```python
from build123d import *

# Parameters (mm, degrees)
BOSS_EXTRUDE1_DEPTH = 22.5
SKETCH2_W           = 5
SKETCH2_H           = 5
CUT_EXTRUDE1_DEPTH  = 10


with BuildPart() as part:
    # Sketch1 → Boss-Extrude1 (new, symmetric)
    with BuildSketch(Plane.XY):
        with BuildLine():
            Line((1.939814393, 10.4209942), (1.904028006, 10.276656915))
            ThreePointArc((1.904028006, 10.276656915), (1.428480454, 9.568373768), (0.609305018, 9.330125797))
            ThreePointArc((0.609305018, 9.330125797), (-0.439609364, 9.339659716), (-1.482990759, 9.231643321))
            ThreePointArc((-1.482990759, 9.231643321), (-2.320923107, 9.391892722), (-2.860897269, 10.052376178))
            Line((-2.860897269, 10.052376178), (-2.910083052, 10.192713899))
            ThreePointArc((-2.910083052, 10.192713899), (-4.572008101, 10.932485624), (-5.212501917, 9.229833356))
            Line((-5.212501917, 9.229833356), (-5.14713766, 9.096261535))
            ThreePointArc((-5.14713766, 9.096261535), (-5.056152588, 8.248009091), (-5.530534536, 7.538944737))
            ThreePointArc((-5.530534536, 7.538944737), (-6.340177854, 6.872018974), (-7.070022774, 6.118600982))
            ThreePointArc((-7.070022774, 6.118600982), (-7.814922522, 5.702746613), (-8.65311731, 5.861617594))
            Line((-8.65311731, 5.861617594), (-8.781003154, 5.937506514))
            ThreePointArc((-8.781003154, 5.937506514), (-10.529627702, 5.435939703), (-9.925830648, 3.719930906))
            Line((-9.925830648, 3.719930906), (-9.789900412, 3.659624288))
            ThreePointArc((-9.789900412, 3.659624288), (-9.174955642, 3.068309294), (-9.082575516, 2.220207648))
            ThreePointArc((-9.082575516, 2.220207648), (-9.274106664, 1.18888418), (-9.348912558, 0.142597243))
            ThreePointArc((-9.348912558, 0.142597243), (-9.652232836, -0.654778014), (-10.396447593, -1.071857007))
            Line((-10.396447593, -1.071857007), (-10.543194291, -1.095926157))
            ThreePointArc((-10.543194291, -1.095926157), (-11.560317477, -2.604142819), (-9.994752906, -3.530568558))
            Line((-9.994752906, -3.530568558), (-9.851859958, -3.489391835))
            ThreePointArc((-9.851859958, -3.489391835), (-9.000694983, -3.547086522), (-8.38477847, -4.137389275))
            ThreePointArc((-8.38477847, -4.137389275), (-7.868577895, -5.050542735), (-7.253342256, -5.900129331))
            ThreePointArc((-7.253342256, -5.900129331), (-6.973156133, -6.705924732), (-7.275164503, -7.503797802))
            Line((-7.275164503, -7.503797802), (-7.372107645, -7.616562799))
            ThreePointArc((-7.372107645, -7.616562799), (-7.181806226, -9.425717974), (-5.3870192, -9.129075755))
            Line((-5.3870192, -9.129075755), (-5.304024738, -9.005682738))
            ThreePointArc((-5.304024738, -9.005682738), (-4.614909109, -8.502761133), (-3.763650392, -8.559055773))
            ThreePointArc((-3.763650392, -8.559055773), (-2.781254079, -8.926764573), (-1.763852499, -9.182119818))
            ThreePointArc((-1.763852499, -9.182119818), (-1.031262177, -9.61929474), (-0.749751088, -10.424628209))
            Line((-0.749751088, -10.424628209), (-0.751529899, -10.573325059))
            ThreePointArc((-0.751529899, -10.573325059), (0.557151975, -11.836894934), (1.74136066, -10.455986948))
            Line((1.74136066, -10.455986948), (1.725622604, -10.308114601))
            ThreePointArc((1.725622604, -10.308114601), (1.930244025, -9.479899312), (2.618531533, -8.975844952))
            ThreePointArc((2.618531533, -8.975844952), (3.60744943, -8.626054058), (4.550963444, -8.167694395))
            ThreePointArc((4.550963444, -8.167694395), (5.393170812, -8.031689832), (6.126479194, -8.467659221))
            Line((6.126479194, -8.467659221), (6.220697038, -8.582711015))
            ThreePointArc((6.220697038, -8.582711015), (8.035412575, -8.709457202), (8.054938514, -6.890425643))
            Line((8.054938514, -6.890425643), (7.947831951, -6.78726508))
            ThreePointArc((7.947831951, -6.78726508), (7.572214528, -6.021287246), (7.775473452, -5.192736523))
            ThreePointArc((7.775473452, -5.192736523), (8.308187259, -4.289116981), (8.736333014, -3.33151399))
            ThreePointArc((8.736333014, -3.33151399), (9.29407924, -2.68596799), (10.136061773, -2.548578376))
            Line((10.136061773, -2.548578376), (10.282190696, -2.5761511))
            ThreePointArc((10.282190696, -2.5761511), (11.753814328, -1.50676765), (10.599521117, -0.100757601))
            Line((10.599521117, -0.100757601), (10.451162399, -0.090578797))
            ThreePointArc((10.451162399, -0.090578797), (9.671061698, 0.254752041), (9.294184928, 1.020111037))
            ThreePointArc((9.294184928, 1.020111037), (9.121431934, 2.0547456), (8.833875273, 3.063518836))
            ThreePointArc((8.833875273, 3.063518836), (8.8461847, 3.916548126), (9.402868399, 4.563010616))
            Line((9.402868399, 4.563010616), (9.532533054, 4.635818545))
            ThreePointArc((9.532533054, 4.635818545), (9.972475727, 6.400955231), (8.184469989, 6.736056042))
            Line((8.184469989, 6.736056042), (8.064277808, 6.648490313))
            ThreePointArc((8.064277808, 6.648490313), (7.244711617, 6.411590018), (6.464043982, 6.755637305))
            ThreePointArc((6.464043982, 6.755637305), (5.666657234, 7.437169878), (4.797949114, 8.025097152))
            ThreePointArc((4.797949114, 8.025097152), (4.259062024, 8.686467846), (4.269968399, 9.539516228))
            Line((4.269968399, 9.539516228), (4.322497253, 9.678637172))
            ThreePointArc((4.322497253, 9.678637172), (3.524904902, 11.313600021), (1.939814393, 10.4209942))
        make_face()
    extrude(amount=BOSS_EXTRUDE1_DEPTH, both=True)

    # Sketch2 → Cut-Extrude1 (cut)
    with BuildSketch(Plane.XY.offset(22.5)):
        with BuildLine():
            Line((-3, -4), (3, -4))
            ThreePointArc((3, -4), (3.535533906, -3.535533906), (4, -3))
            Line((4, -3), (4, 3))
            ThreePointArc((4, 3), (3.535533906, 3.535533906), (3, 4))
            Line((3, 4), (-3, 4))
            ThreePointArc((-3, 4), (-3.535533906, 3.535533906), (-4, 3))
            Line((-4, 3), (-4, -3))
            ThreePointArc((-4, -3), (-3.535533906, -3.535533906), (-3, -4))
        make_face()
        Rectangle(SKETCH2_W, SKETCH2_H, mode=Mode.SUBTRACT)
    cut_extrude1 = extrude(amount=-CUT_EXTRUDE1_DEPTH, mode=Mode.SUBTRACT)

    # Mirror1: Cut-Extrude1 across plane
    add(cut_extrude1.mirror(Plane.XY), mode=Mode.SUBTRACT)


solid = part.part
```
Could you check a few things on this model? Use its own coordinates, in mm. A direction names the side the tool comes from. Round coordinates to 2 decimals unless told otherwise and drop trailing zeros. Loops run counter-clockwise (first coordinate to the right, second up) from the corner with the lowest first, then second, coordinate; pieces in that order, holes last. Notation, with made-up numbers: M 44.5,-3 L 97.5,-3 A24 cw 97.5,19 Z; hole C 59,-35 d3. An arc over 180 degrees is marked long. Answer as CSV lines item,"result".
1) If I drill on probe 1 along Y at (x, z) = (-3.75, -14); probe 2 along X at (y, z) = (1, 15); probe 3 along X at (y, z) = (2.25, -13.5), over which ranges is the centre line in solid material (lowest first)?
From the geometry:
probe 1,"-8.57 to -3.31, 3.31 to 10.98"
probe 2,"-9.3 to -4, -2.5 to 2.5, 4 to 9.3"
probe 3,"-9.08 to -4, -2.5 to 2.5, 4 to 9.08"
2) Which directions (+Z, -Z, +X, -X, +Y, -Y) give clear straight access to the entire face, cutting with the end or side of a thin tool? Please do faces 4 (the flat face through (-2.5, 0, -18)), 5 (the cylindrical face through (-7.2, -9.41, 0.32)), 6 (the flat face through (5, 0, -22.5)), 7 (the flat face through (0, -2.5, 18)), 8 (the cylindrical face through (9.68, 0.246, 0.315)).
From the geometry:
face 4,"-Z"
face 5,"+Z, -Z"
face 6,"-Z, +X, -X, +Y, -Y"
face 7,"+Z"
face 8,"+Z, -Z, +X"
3) Imagine slicing it at A-A on z = 13. Count the separate pieces of the cut face and the enclosed holes in it, and give its area (3 significant figures).
From the geometry:
separate pieces,"2"
enclosed holes,"1"
area,"292 mm^2"
4) Imagine slicing it at B-B on x = 7. List the corners of the cut face in (y, z) for me, and give its area (3 significant figures).
From the geometry:
outline,"M -9.03,-22.5 L 6.45,-22.5 L 6.45,22.5 L -9.03,22.5 Z"
area,"697 mm^2"
5) For pin 1 Ø6 at (x, z) = (7, 10) entering from -Y; pin 2 Ø3 at (y, z) = (1, -19) entering from -X; pin 3 Ø2 at (y, z) = (-2.5, 17) entering from +X, each with a flat end and sliding along its axis, tell me the tip position at first contact or that it passes through.
From the geometry:
pin 1,"y = -9.04"
pin 2,"x = -9.54"
pin 3,"x = 11.75"
6) We'd pull the mould along Y, two halves only. Please class faces 1 (the cylindrical face through (7.26, 6.41, 0.32)), 2 (the cylindrical face through (9.988, 6.377, 0.315)), 3 (the cylindrical face through (-4.6, -8.5, 0.3)): released by +Y, released by -Y, zero draft, split by the parting line, or undercut.
From the geometry:
face 1,"released by +Y"
face 2,"undercut"
face 3,"released by -Y"
